Build history of the part. All positions in model axes, mm. Round coordinates to 2 decimals unless told otherwise and drop trailing zeros. Loops run counter-clockwise (first coordinate to the right, second up) from the corner with the lowest first, then second, coordinate; pieces in that order, holes last. Notation, with made-up numbers: (57.25, 18) - (96.25, 18) arc R22 ccw to (96.25, 46) - close; hole circle Ø6 at (-23, 40.5). An arc over 180 degrees is marked (long way). Use one line per item in the form item = value. Start each with the question number.
Q1. Drill centre lines: line 1 (Z direction, x = -53.5, y = -25.4); line 2 (Y direction, x = -38, z = 34.5); line 3 (Z direction, x = -58, y = -25). Where is each one in solid material? Low to high.
Q2. Saw through at B-B (y = -25.4). Give the cut face in (x, z).
Q3. Saw through at C-C (x = -59.5). Give the cut face in (y, z) (3 decimals), then the cut area to 3 significant figures.
Q4. Saw through at A-A (y = -6.35). Give the cut face in (x, z), then the cut area to 3 significant figures.
Q5. Mould opens along Z. For faces 1 (the face through (-53, -25, 24.672)), 2 (the face through (-52.25, -39.19, 43.34)), 3 (the face through (-36.594, -25, 68)), 4 (the face through (-52.246, -22.467, 74.256)) say: released by +Z, released by -Z, zero draft, split by the parting line, or undercut.
```python
from build123d import *

# Parameters (mm, degrees)
F0_W     = 31.75
F0_H     = 88.9
F1_DEPTH = 50.8
F2_R     = 3.175
F3_DEPTH = 76.2
F4_R     = 3.175
F5_DEPTH = 25.4
F6_DEPTH = 38.1


with BuildPart() as f1:
    # F0 (on Front) → F1 (new body)
    with BuildSketch(Plane.XZ):
        with Locations((-52.468664, 69.122105)):
            Rectangle(F0_W, F0_H)
    extrude(amount=F1_DEPTH)

    # F2 (on face) → F3 (cut)
    with BuildSketch(Plane.YZ.offset(-36.593664)):
        with Locations((-25.4, 75.472105)):
            Circle(F2_R)
        with Locations((-25.4, 32.292105)):
            Circle(F2_R)
        with Locations((-6.35, 37.372105)):
            Circle(F2_R)
    extrude(amount=-F3_DEPTH, mode=Mode.SUBTRACT)

    # F4 (on face) → F5 (cut)
    with BuildSketch(Plane.YZ.offset(-36.593664)):
        with Locations((-36.850315, 41.194014)):
            Circle(F4_R)
    extrude(amount=-F5_DEPTH, mode=Mode.SUBTRACT)

    # F4 (on face) → F6 (cut)
    with BuildSketch(Plane.YZ.offset(-36.593664)):
        with Locations((-36.850315, 41.194014)):
            Circle(F4_R)
    extrude(amount=-F6_DEPTH, mode=Mode.SUBTRACT)


solid = f1.part
```
Report:
q1.line_1 = 24.67 to 29.12, 35.47 to 72.3, 78.65 to 113.57
q1.line_2 = -50.8 to -27.68, -23.12 to -7.7, -5 to 0
q1.line_3 = 24.67 to 29.14, 35.44 to 72.32, 78.62 to 113.57
q2.outline = (-68.34, 24.67) - (-36.59, 24.67) - (-36.59, 29.12) - (-68.34, 29.12) - close; (-68.34, 35.47) - (-36.59, 35.47) - (-36.59, 72.3) - (-68.34, 72.3) - close; (-68.34, 78.65) - (-36.59, 78.65) - (-36.59, 113.57) - (-68.34, 113.57) - close
q3.outline = (-50.8, 24.672) - (0, 24.672) - (0, 113.572) - (-50.8, 113.572) - close; hole circle Ø6.35 at (-36.85, 41.194); hole circle Ø6.35 at (-25.4, 32.292); hole circle Ø6.35 at (-25.4, 75.472); hole circle Ø6.35 at (-6.35, 37.372)
q3.area = 4,390 mm²
q4.outline = (-68.34, 24.67) - (-36.59, 24.67) - (-36.59, 34.2) - (-68.34, 34.2) - close; (-68.34, 40.55) - (-36.59, 40.55) - (-36.59, 113.57) - (-68.34, 113.57) - close
q4.area = 2,620 mm²
q5.face_1 = released by -Z
q5.face_2 = undercut
q5.face_3 = zero draft
q5.face_4 = undercut
